Verification items for the finished model (mm, model axes). A direction names the side the tool comes from. Give positions to 0.01 mm unless a question says otherwise; leave off trailing zeros. Write each loop counter-clockwise with the first axis right and the second up, starting at its lowest first coordinate (ties: lowest second). Pieces come first, ordered by that corner, then holes.
from build123d import *

# Parameters (mm, degrees)
BOSS_EXTRUDE1_DEPTH     = 4.65
CUT_EXTRUDE4_DEPTH      = 22.226045322
CUT_EXTRUDE4_DEPTH_BACK = 22.226045322
SKETCH3_W               = 3.05
SKETCH3_H               = 2.5
SKETCH4_R               = 0.75
CUT_EXTRUDE1_DEPTH      = 10


with BuildPart() as part:
    # Sketch1 → Boss-Extrude1 (new, symmetric)
    with BuildSketch(Plane.XY):
        Polygon((-4.75, 11.5), (-4.75, 16), (-6.65, 16), (-6.65, 11.5), (-13.15, 11.5), (-13.15, -9.5), (-13.15, -11.5), (-10.95, -11.5), (-6.65, -11.5), (-6.65, -16), (-4.75, -16), (-4.75, -11.5), (13.15, -11.5), (13.15, 11.5), align=None)
    extrude(amount=BOSS_EXTRUDE1_DEPTH, both=True)

    # Sketch7 → Cut-Extrude4 (cut, two sides: drawn at the far end of the back side and taken through both)
    with BuildSketch(Plane.XY.offset(-CUT_EXTRUDE4_DEPTH_BACK)):
        Polygon((-11.251215972, -10.366937752), (-13.15, -9.5), (-13.15, -11.5), (-10.95, -11.5), align=None)
    extrude(amount=CUT_EXTRUDE4_DEPTH + CUT_EXTRUDE4_DEPTH_BACK, mode=Mode.SUBTRACT)

    # Sketch3 → Revolve1 (revolve)
    with BuildSketch(Plane.XY, mode=Mode.PRIVATE) as revolve1_sk:
        with Locations((-14.675, 8.05)):
            Rectangle(SKETCH3_W, SKETCH3_H)
    revolve(revolve1_sk.sketch.rotate(Axis((-13.15, 6.8, 0), (-1, 0, 0)), 90), axis=Axis((-13.15, 6.8, 0), (-1, 0, 0)))

    # Sketch4 → Cut-Extrude1 (cut)
    with BuildSketch(Plane.ZY.offset(6.65)):
        with Locations(Location((0, 14.4, 0), (0, 0, 270))):
            Circle(SKETCH4_R)
        with Locations(Location((0, -14.4, 0), (0, 0, 270))):
            Circle(SKETCH4_R)
    extrude(amount=-CUT_EXTRUDE1_DEPTH, mode=Mode.SUBTRACT)


solid = part.part
Item 1: Release check for a two-part mould opening along Z. For faces 1 (the face through (-6, -16, 0)), 2 (the face through (-5.713, 13.685, 0.225)), 3 (the face through (0, 0, -4.65)) record: released by +Z, released by -Z, zero draft, split by the parting line, or undercut.
Answer key:
face 1: zero draft
face 2: undercut
face 3: released by -Z
Item 2: Sectioned sample at D-D on y = 6.8. Record the cut outline in (x, z), then the cut area to 3 significant figures.
Answer key:
outline: (-16.2, -2.5) - (-13.15, -2.5) - (-13.15, -4.65) - (13.15, -4.65) - (13.15, 4.65) - (-13.15, 4.65) - (-13.15, 2.5) - (-16.2, 2.5) - close
area: 260 mm2
Item 3: Set-up check for faces 4 (the face through (-4.75, 13, 0)), 5 (the face through (-9, -11.5, 0)), 6 (the face through (4, -11.5, 0)), 7 (the face through (-10, 11.5, 0)): record each of +Z, -Z, +X, -X, +Y, -Y from which the full face is reachable in a straight line by a thin tool's end or side.
Answer key:
face 4: +Z, -Z, +X, +Y
face 5: +Z, -Z, -X, -Y
face 6: +Z, -Z, +X, -Y
face 7: +Z, -Z, -X, +Y
Item 4: Sectioned sample at B-B on y = -14.4. Record the cut outline in (x, z), then the cut area to 3 significant figures.
Answer key:
outline: (-6.65, -4.65) - (-4.75, -4.65) - (-4.75, -0.75) - (-6.65, -0.75) - close; (-6.65, 0.75) - (-4.75, 0.75) - (-4.75, 4.65) - (-6.65, 4.65) - close
area: 14.8 mm2
Item 5: Sectioned sample at C-C on z = -3. Record the cut outline in (x, y), then the cut area to 3 significant figures.
Answer key:
outline: (-13.15, -9.5) - (-11.25, -10.37) - (-10.95, -11.5) - (-6.65, -11.5) - (-6.65, -16) - (-4.75, -16) - (-4.75, -11.5) - (13.15, -11.5) - (13.15, 11.5) - (-4.75, 11.5) - (-4.75, 16) - (-6.65, 16) - (-6.65, 11.5) - (-13.15, 11.5) - close
area: 619 mm2
Item 6: Depth check by flat-ended pin: pin 1 (2 mm diameter, centred on y = 14.5, z = -1.5, fed in from -X); pin 2 (2 mm diameter, centred on x = -11.5, z = -2, fed in from +Y); pin 3 (3.5 mm diameter, centred on y = 13.5, z = 2.5, fed in from +X); pin 4 (1.4 mm diameter, centred on y = 14.4, z = 0, fed in from +X). Enter the tip coordinate at first touch or a pass-through.
Answer key:
pin 1: stops at x = -6.65
pin 2: stops at y = 11.5
pin 3: stops at x = -4.75
pin 4: passes through
Item 7: Sectioned sample at A-A on z = 0. Record the cut outline in (x, y), then the cut area to 3 significant figures.
Answer key:
outline: (-16.2, 4.3) - (-13.15, 4.3) - (-13.15, -9.5) - (-11.25, -10.37) - (-10.95, -11.5) - (-6.65, -11.5) - (-6.65, -13.65) - (-4.75, -13.65) - (-4.75, -11.5) - (13.15, -11.5) - (13.15, 11.5) - (-4.75, 11.5) - (-4.75, 13.65) - (-6.65, 13.65) - (-6.65, 11.5) - (-13.15, 11.5) - (-13.15, 9.3) - (-16.2, 9.3) - close; (-6.65, -16) - (-4.75, -16) - (-4.75, -15.15) - (-6.65, -15.15) - close; (-6.65, 15.15) - (-4.75, 15.15) - (-4.75, 16) - (-6.65, 16) - close
area: 628 mm2
Item 8: Scan lines: line 1 along Z through (x, y) = (-5.2, 14.4); line 2 along X through (y, z) = (7.5, 3.25); line 3 along X through (y, z) = (12.5, -3.5). Record each from-to range of solid material in increasing order.
Answer key:
line 1: z = -4.65 to -0.75, 0.75 to 4.65
line 2: x = -13.15 to 13.15
line 3: x = -6.65 to -4.75
